The model under review builds one solid part; all positions refer to its coordinate system, in mm. Round coordinates to 2 decimals unless told otherwise and drop trailing zeros. Write each loop counter-clockwise with the first axis right and the second up, starting at its lowest first coordinate (ties: lowest second). Pieces come first, ordered by that corner, then holes. Notation, with made-up numbers: (-3, 82) -> (49, 82) arc R17 ccw to (49, 114) -> close; hole circle Ø11 at (60, 43.25). An arc over 180 degrees is marked (long way). Return JSON: item names as keys, results as strings. Group by question number.
1. Take a section at D-D, the plane y = -14. Write out the cut boundary in (x, z), then the cut area to 3 significant figures.
2. Clearance check with a flat-ended pin moving along its axis: P1, Ø0.8, axis at x = -6.5, z = -1.5, coming from the -Y side. State where the tip first meets the part, or that it passes through.
3. Mouldability with a two-part tool opening along X and no side actions: class faces 1 (the flat face through (-19.16, 19.08, -1.25)), 2 (the flat face through (24, 3, 0)), 3 (the cylindrical face through (30.453, 15.865, -1.252)) as pulls with the +X half, pulls with the -X half, needs draft (parallel to the pull), parting line crosses it, or undercut.
4. For line 1 along X through (y, z) = (-0.5, -1.95); line 2 along X through (y, z) = (6, -2.25) (3 decimals); line 3 along Y through (x, z) = (0, -0.7) (1 decimal), list the stretches that pass through material, from the lowest coordinate up. Write a range as from..to.
5. Take a section at A-A, the plane x = 0. Write out the cut boundary in (y, z) (1 decimal).
6. Take a section at C-C, the plane z = -1.5. Give the number of separate pieces and of enclosed holes in the cut face, then the cut area to 3 significant figures.
7. Take a section at B-B, the plane y = -9. Write out the cut boundary in (x, z), then the cut area to 3 significant figures.
from build123d import *

# Parameters (mm, degrees)
MODEL_R             = 2.032
MODEL_R_2           = 3.2639
MODEL_R_3           = 15.24
MODEL_R_4           = 18.415
BOSS_EXTRUDE1_DEPTH = 2.54


with BuildPart() as part:
    # Model → Boss-Extrude1 (new body)
    with BuildSketch(Plane.XY):
        Polygon((23.89577784, 19.950554749), (20.085777841, 19.950499596), (18.29294446, 19.955499209), (-18.28305554, 19.955499209), (-20.06105554, 18.177499209), (-20.06105554, -18.398500791), (-18.28305554, -20.176500791), (18.29294446, -20.176500791), (20.066, -20.181445251), (23.876, -20.181445251), (60.660238165, -20.181445251), (62.438238165, -18.413722656), (62.418460324, 18.066456797), (60.640460324, 19.950554749), align=None)
        with Locations((-14.99997, -14.99997)):
            Circle(MODEL_R, mode=Mode.SUBTRACT)
        with Locations((14.99997, -14.99997)):
            Circle(MODEL_R, mode=Mode.SUBTRACT)
        with Locations((27.358298165, -15.115415251)):
            Circle(MODEL_R_2, mode=Mode.SUBTRACT)
        with Locations((57.358238165, -15.115415251)):
            Circle(MODEL_R_2, mode=Mode.SUBTRACT)
        with Locations((42.268119082, -0.17363293)):
            Circle(MODEL_R_3, mode=Mode.SUBTRACT)
        Circle(MODEL_R_4, mode=Mode.SUBTRACT)
        with Locations((-14.99997, 14.99997)):
            Circle(MODEL_R, mode=Mode.SUBTRACT)
        with Locations((14.99997, 14.99997)):
            Circle(MODEL_R, mode=Mode.SUBTRACT)
        with Locations((27.340244675, 14.884524749)):
            Circle(MODEL_R_2, mode=Mode.SUBTRACT)
        with Locations((57.340184675, 14.884519317)):
            Circle(MODEL_R_2, mode=Mode.SUBTRACT)
    extrude(amount=-BOSS_EXTRUDE1_DEPTH)


solid = part.part
Output:
{
 "1": {"outline": "(-20.06, -2.54) -> (-16.77, -2.54) -> (-16.77, 0) -> (-20.06, 0) -> close; (-13.23, -2.54) -> (-11.96, -2.54) -> (-11.96, 0) -> (-13.23, 0) -> close; (11.96, -2.54) -> (13.23, -2.54) -> (13.23, 0) -> (11.96, 0) -> close; (16.77, -2.54) -> (24.29, -2.54) -> (24.29, 0) -> (16.77, 0) -> close; (30.43, -2.54) -> (35.86, -2.54) -> (35.86, 0) -> (30.43, 0) -> close; (48.68, -2.54) -> (54.29, -2.54) -> (54.29, 0) -> (48.68, 0) -> close; (60.43, -2.54) -> (62.44, -2.54) -> (62.44, 0) -> (60.43, 0) -> close", "area": "67.1 mm^2"},
 "2": {"P1": "stops at y = -20.18"},
 "3": {"face 1": "pulls with the -X half", "face 2": "needs draft", "face 3": "undercut"},
 "4": {"line 1": "x = -20.06..-18.41, 18.41..27.03, 57.5..62.43", "line 2": "x = -20.061..-17.41, 17.41..28.335, 56.202..62.425", "line 3": "y = -20.2..-18.4, 18.4..20"},
 "5": {"outline": "(-20.2, -2.5) -> (-18.4, -2.5) -> (-18.4, 0) -> (-20.2, 0) -> close; (18.4, -2.5) -> (20, -2.5) -> (20, 0) -> (18.4, 0) -> close"},
 "6": {"separate pieces": "1", "enclosed holes": "10", "area": "1,320 mm^2"},
 "7": {"outline": "(-20.06, -2.54) -> (-16.07, -2.54) -> (-16.07, 0) -> (-20.06, 0) -> close; (16.07, -2.54) -> (29.84, -2.54) -> (29.84, 0) -> (16.07, 0) -> close; (54.69, -2.54) -> (62.43, -2.54) -> (62.43, 0) -> (54.69, 0) -> close", "area": "64.8 mm^2"}
}
